Autodesk Inventor part; units mm, degrees
ref_plane "Work Plane1" through (0, 0, 57.15) normal (0, 0, -1) x (-1, 0, 0)
ref_plane "YZ Plane" through (0, 0, 0) normal (1, 0, 0) x (0, 1, 0)
ref_plane "XZ Plane" through (0, 0, 0) normal (0, 1, 0) x (-1, 0, 0)
sketch "Sketch1" plane through (0, 0, 0) normal (0, 0, 1) x (1, 0, 0)
  arc A0 (-12.6587, -1.0228) -> (12.6587, -1.0228) centre (0, 0) ccw
  line L0 (0, 0) -> (0, -38.1)
  line L1 (0, -38.1) -> (-9.663, -38.1)
  line L2 (-9.663, -38.1) -> (-12.6587, -1.0228)
  line L3 (0, -38.1) -> (9.663, -38.1)
  line L4 (9.663, -38.1) -> (12.6587, -1.0228)
  dimension "d0" = 25.4
  dimension "d1" = 38.1
  dimension "d2" = 9.663
  dimension "d3" = 9.663
extrude "Extrusion1" add sketch "Sketch1" along normal blind 114.3
shell "Shell1" thickness 2.54 removed faces 1 at (-12.5308, -2.0661, 76.2)
sketch "Sketch2" plane through (-9.5133, -8.4135, 111.76) normal (0.9968, 0.0805, 0) x (0, 0, -1)
  line L0 (109.22, 0) -> (109.22, -27.235)
  line L1 (0, 0) -> (109.22, 0)
  line L2 (0, 0) -> (0, -27.235)
  line L3 (109.22, -27.235) -> (0, -27.235)
  line L4 (106.68, -2.54) -> (106.68, -24.695)
  line L5 (106.68, -24.695) -> (2.54, -24.695)
  line L6 (2.54, -24.695) -> (2.54, -2.54)
  line L7 (2.54, -2.54) -> (106.68, -2.54)
  point P0 (111.76, 7.62)
  dimension "d9" = 2.54
sketch "Sketch3" plane through (-9.663, -38.1, 0) normal (-0.9968, -0.0805, 0) x (0, 0, 1)
  line L0 (2.54, 29.578) -> (2.54, 2.3431)
  line L1 (111.76, 29.578) -> (2.54, 29.578)
  line L2 (111.76, 29.578) -> (111.76, 2.3431)
  line L3 (2.54, 2.3431) -> (111.76, 2.3431)
  point P0 (0, 37.198)
extrude "Extrusion2" cut sketch "Sketch3" against normal blind 1.27
extrude "Extrusion3" cut sketch "Sketch2" against normal blind 1.27 contours L4 L5 L6 L7
mirror "Mirror1" about plane through (0, 0, 0) normal (1, 0, 0) of "Extrusion3", "Extrusion2"
sketch "Sketch4" plane through (-7.32, -35.56, 2.54) normal (0, 1, 0) x (1, 0, 0)
  line L0 (16.8333, -109.22) -> (-2.1933, -109.22)
  line L1 (7.32, -109.22) -> (6.431, -109.22)
  line L2 (6.431, -109.22) -> (6.431, -106.172)
  line L3 (6.431, -106.172) -> (3.383, -106.172)
  line L4 (3.383, -106.172) -> (3.383, -109.22)
  line L5 (-2.1933, -109.22) -> (16.8333, -109.22)
  line L6 (7.32, -109.22) -> (8.209, -109.22)
  line L7 (8.209, -109.22) -> (8.209, -106.172)
  line L8 (8.209, -106.172) -> (11.257, -106.172)
  line L9 (11.257, -106.172) -> (11.257, -109.22)
  point P0 (7.32, 2.54)
  dimension "d12" = 0.889
  dimension "d13" = 3.048
  dimension "d14" = 3.048
extrude "Extrusion4" add sketch "Sketch4" along normal blind 26.67
ref_plane "Work Plane1" through (0, 0, 57.15) normal (0, 0, -1) x (-1, 0, 0)
mirror "Mirror2" about plane through (0, 0, 57.15) normal (0, 0, -1) of "Extrusion4"
sketch "Sketch6" plane through (0, 0, 0) normal (0, 0, -1) x (-1, 0, 0)
  arc A0 (-12.6587, -1.0228) -> (12.6587, -1.0228) centre (0, 0) ccw
  line L0 (-12.6587, -1.0228) -> (12.6587, -1.0228)
extrude "Extrusion6" cut sketch "Sketch6" against normal blind 304.8
sketch "Sketch7" plane through (0, 0, 0) normal (0, 0, -1) x (-1, 0, 0)
  line L0 (-8.8842, -16.2006) -> (-9.5133, -8.4135)
  line L1 (-3.937, -12.0744) -> (-3.937, -16.2006)
  line L2 (-8.8842, -16.2006) -> (-3.937, -16.2006)
  line L3 (-3.937, -16.2006) -> (-3.937, -12.0744)
  arc A0 (-9.5133, -8.4135) -> (-3.937, -12.0744) centre (0, 0) ccw
properties part number "Tractive Light Mount"
Work out the finished part from the listing and answer in its coordinate system (mm). A direction names the side the tool comes from. Give positions to 0.01 mm unless a question says otherwise; leave off trailing zeros. Write each loop counter-clockwise with the first axis right and the second up, starting at its lowest first coordinate (ties: lowest second). Pieces come first, ordered by that corner, then holes.
(1) The part is cut by section A-A on z = 91.5. Write down the section's boundary in (x, y).
Final values:
outline: (-12.66, -1.02) - (-12.05, -8.62) - (-10.78, -8.52) - (-10.57, -11.05) - (-9.31, -10.95) - (-9.51, -8.41) arc R12.7 cw to start; (-9.85, -35.76) - (-9.66, -38.1) - (9.66, -38.1) - (9.85, -35.76) - (8.58, -35.66) - (8.79, -33.13) - (7.52, -33.03) - (7.32, -35.56) - (-7.32, -35.56) - (-7.52, -33.03) - (-8.79, -33.13) - (-8.58, -35.66) - close; (9.31, -10.95) - (10.57, -11.05) - (10.78, -8.52) - (12.05, -8.62) - (12.66, -1.02) arc R12.7 cw to (9.51, -8.41) - close
(2) Flat-ended cylindrical pins translate along their axes: pin 1 Ø6 at (x, y) = (1, -12) entering from -Z; pin 2 Ø2 at (x, z) = (-2, 74.5) entering from +Y; pin 3 Ø2.5 at (y, z) = (-21, 3.5) entering from +X; pin 4 Ø5 at (y, z) = (-8, 17.5) entering from +X. Find the tip coordinate at first contact, or state that the pin passes through.
Final values:
pin 1: stops at z = 0
pin 2: stops at y = -35.56
pin 3: stops at x = 11.11
pin 4: stops at x = 12.3
(3) Which of the six approach directions +Z, -Z, +X, -X, +Y, -Y give full straight-line access (tool end or side, diameter ignored) to faces 4 (the flat face through (-0.889, -24, 4)), 5 (the flat face through (12.152, -7.289, 56.883)), 6 (the flat face through (10, -22, 2.54)), 7 (the flat face through (-10, -22, 111.76))?
Final values:
face 4: +Y
face 5: +Z, -Z, +X, -Y
face 6: +X
face 7: -X
(4) The part is cut by section D-D on x = -2.25. Write down the section's boundary in (y, z), plus the area to 3 significant figures.
Final values:
outline: (-38.1, 0) - (-12.5, 0) - (-12.5, 5.59) - (-35.56, 5.59) - (-35.56, 108.71) - (-12.5, 108.71) - (-12.5, 114.3) - (-38.1, 114.3) - close
area: 548 mm2
(5) The part is cut by section C-C on x = 5.25. Write down the section's boundary in (y, z).
Final values:
outline: (-38.1, 0) - (-11.56, 0) - (-11.56, 2.54) - (-35.56, 2.54) - (-35.56, 111.76) - (-11.56, 111.76) - (-11.56, 114.3) - (-38.1, 114.3) - close
(6) The mould has two halves that part along Y. Classify faces 1 (the flat face through (6, -22, 111.76)), 2 (the flat face through (-10, -22, 2.54)), 3 (the flat face through (0, -38.1, 56)): pulls with the +Y half, pulls with the -Y half, needs draft (parallel to the pull), parting line crosses it, or undercut.
Final values:
face 1: needs draft
face 2: undercut
face 3: pulls with the -Y half
(7) The part is cut by section B-B on y = -2.5. Write down the section's boundary in (x, z), plus the area to 3 significant figures.
Final values:
outline: (-12.54, 0) - (-12.45, 0) - (-12.45, 114.3) - (-12.54, 114.3) - close; (12.45, 0) - (12.54, 0) - (12.54, 114.3) - (12.45, 114.3) - close
area: 20.1 mm2
(8) Straight lines are drawn through the part: line 1 (Z direction, x = -5, y = -22.5); line 2 (Z direction, x = 2.75, y = -35); line 3 (X direction, y = -35.5, z = 45.5). For each, find the intervals that lie inside material, in ascending order.
Final values:
line 1: z = 0 to 2.54, 111.76 to 114.3
line 2: z = 0 to 5.59, 108.71 to 114.3
line 3: x = -8.6 to -7.32, 7.32 to 8.6
